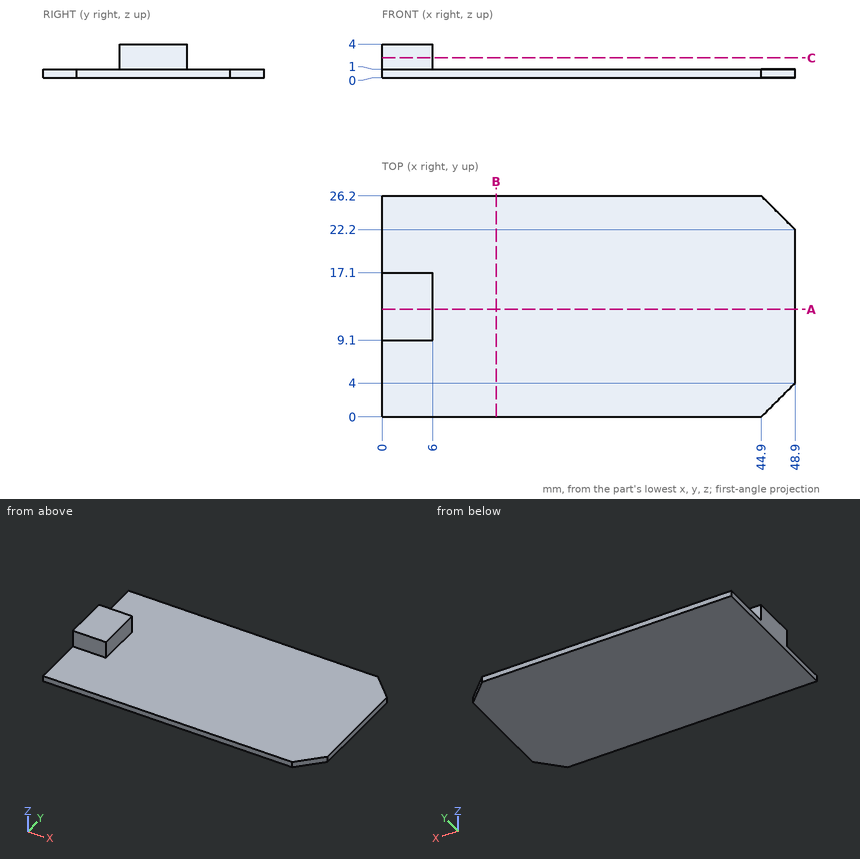
The figure shows three views and two pictorial views of one solid part (mm, origin at its lowest corner). Answer the questions. Coordinates: 2 decimals unless noted, no trailing zeros. Write each loop counter-clockwise with the first axis right and the second up, starting at its lowest first coordinate (ties: lowest second). Pieces come first, ordered by that corner, then holes.
1. Flat-ended cylindrical pins translate along their axes: pin 1 (12 mm diameter, centred on x = 43, y = 10, fed in from -Z); pin 2 (12 mm diameter, centred on x = 25.5, y = 7.5, fed in from +Z); pin 3 (0.9 mm diameter, centred on y = 13.5, z = 2, fed in from +X); pin 4 (1.5 mm diameter, centred on x = 3, z = 2.5, fed in from +Y). Find the tip coordinate at first contact, or state that the pin passes through.
Results list:
pin 1: stops at z = 0
pin 2: stops at z = 1
pin 3: stops at x = 6
pin 4: stops at y = 17.1
2. The part is cut by section B-B, the plane x = 13.5. Write down the section's boundary in (y, z), and give its area (3 significant figures).
Results list:
outline: (0, 0) - (26.2, 0) - (26.2, 1) - (0, 1) - close
area: 26.2 mm2
3. The part is cut by section A-A, the plane y = 12.75. Write down the section's boundary in (x, z).
Results list:
outline: (0, 0) - (48.9, 0) - (48.9, 1) - (6, 1) - (6, 4) - (0, 4) - close
4. The part is cut by section C-C, the plane z = 2.35. Write down the section's boundary in (x, y).
Results list:
outline: (0, 9.1) - (6, 9.1) - (6, 17.1) - (0, 17.1) - close
5. Consider line 1 along X through (y, z) = (13.75, 2.4); line 2 along Z through (x, y) = (33, 12.5); line 3 along Y through (x, z) = (5, 2.15). Determine where each line is inside the solid, lowest interval first.
Results list:
line 1: x = 0 to 6
line 2: z = 0 to 1
line 3: y = 9.1 to 17.1
